from build123d import *

# Parameters (mm, degrees)
SKETCH1_W           = 101.6
SKETCH1_H           = 101.6
SKETCH1_R           = 6.5
SKETCH1_R_2         = 1.5
SKETCH1_R_3         = 3.175
SKETCH1_R_4         = 4
SKETCH1_R_5         = 2.0828
BOSS_EXTRUDE1_DEPTH = 5.9944


with BuildPart() as part:
    # Sketch1 → Boss-Extrude1 (new body)
    with BuildSketch(Plane.XY):
        with Locations((50.8, 50.8)):
            Rectangle(SKETCH1_W, SKETCH1_H)
        with Locations(Location((76.2, 57.8, 0), (0, 0, 180))):
            Circle(SKETCH1_R, mode=Mode.SUBTRACT)
        with Locations(Location((60.7, 50.8, 0), (0, 0, 180))):
            Circle(SKETCH1_R_2, mode=Mode.SUBTRACT)
        with Locations(Location((91.7, 50.8, 0), (0, 0, 180))):
            Circle(SKETCH1_R_2, mode=Mode.SUBTRACT)
        with Locations(Location((83.95, 37.376606241, 0), (0, 0, 180))):
            Circle(SKETCH1_R_2, mode=Mode.SUBTRACT)
        with Locations(Location((68.45, 37.376606241, 0), (0, 0, 180))):
            Circle(SKETCH1_R_2, mode=Mode.SUBTRACT)
        with Locations(Location((68.45, 64.223393759, 0), (0, 0, 180))):
            Circle(SKETCH1_R_2, mode=Mode.SUBTRACT)
        with Locations(Location((83.95, 64.223393759, 0), (0, 0, 180))):
            Circle(SKETCH1_R_2, mode=Mode.SUBTRACT)
        with Locations(Location((12.7, 88.9, 0), (0, 0, 180))):
            Circle(SKETCH1_R_3, mode=Mode.SUBTRACT)
        with Locations(Location((88.9, 88.9, 0), (0, 0, 180))):
            Circle(SKETCH1_R_3, mode=Mode.SUBTRACT)
        with Locations(Location((25.4, 57.8, 0), (0, 0, 180))):
            Circle(SKETCH1_R_4, mode=Mode.SUBTRACT)
        with Locations(Location((15.875, 67.325, 0), (0, 0, 180))):
            Circle(SKETCH1_R_5, mode=Mode.SUBTRACT)
        with Locations(Location((34.925, 67.325, 0), (0, 0, 180))):
            Circle(SKETCH1_R_5, mode=Mode.SUBTRACT)
        with Locations(Location((34.925, 48.275, 0), (0, 0, 180))):
            Circle(SKETCH1_R_5, mode=Mode.SUBTRACT)
        with Locations(Location((15.875, 48.275, 0), (0, 0, 180))):
            Circle(SKETCH1_R_5, mode=Mode.SUBTRACT)
        with Locations(Location((50.8, 88.9, 0), (0, 0, 180))):
            Circle(SKETCH1_R_3, mode=Mode.SUBTRACT)
        with Locations(Location((50.8, 25.4, 0), (0, 0, 180))):
            Circle(SKETCH1_R_3, mode=Mode.SUBTRACT)
        with Locations(Location((50.8, 12.7, 0), (0, 0, 180))):
            Circle(SKETCH1_R_3, mode=Mode.SUBTRACT)
    extrude(amount=BOSS_EXTRUDE1_DEPTH)


solid = part.part
CAD build for the part. Positions are in the model's coordinates, mm. Round coordinates to 2 decimals unless told otherwise and drop trailing zeros. Write each loop counter-clockwise with the first axis right and the second up, starting at its lowest first coordinate (ties: lowest second). Pieces come first, ordered by that corner, then holes. Notation, with made-up numbers: (82.25, -33.5) -> (88.25, -33.5) arc R28 cw to (88.25, -1.5) -> close; hole circle Ø3 at (47, 81). An arc over 180 degrees is marked (long way). Answer as a JSON object with one key per item and string values.
(1) Band-saw the part on D-D, the plane x = 50.8. List the corners of the cut face in (y, z) (3 decimals), then the cut area to 3 significant figures.
Reported:
{"outline": "(0, 0) -> (9.525, 0) -> (9.525, 5.994) -> (0, 5.994) -> close; (15.875, 0) -> (22.225, 0) -> (22.225, 5.994) -> (15.875, 5.994) -> close; (28.575, 0) -> (85.725, 0) -> (85.725, 5.994) -> (28.575, 5.994) -> close; (92.075, 0) -> (101.6, 0) -> (101.6, 5.994) -> (92.075, 5.994) -> close", "area": "495 mm^2"}
(2) Two-plate mould, pull along X, no slides. Class faces 1 (the face through (101.6, 50, 3)), 2 (the face through (50, 52, 5.994)), 3 (the face through (67.76, 38.71, 2.96)), 4 (the face through (32.94, 47.65, 2.96)): +X half, -X half, draft (parallel to the pull), parting line (faces both ways), or undercut.
Reported:
{"face 1": "+X half", "face 2": "draft", "face 3": "undercut", "face 4": "undercut"}
(3) Band-saw the part on C-C, the plane y = 88.9. List the corners of the cut face in (x, z) (3 decimals), then the cut area to 3 significant figures.
Reported:
{"outline": "(0, 0) -> (9.525, 0) -> (9.525, 5.994) -> (0, 5.994) -> close; (15.875, 0) -> (47.625, 0) -> (47.625, 5.994) -> (15.875, 5.994) -> close; (53.975, 0) -> (85.725, 0) -> (85.725, 5.994) -> (53.975, 5.994) -> close; (92.075, 0) -> (101.6, 0) -> (101.6, 5.994) -> (92.075, 5.994) -> close", "area": "495 mm^2"}
(4) Band-saw the part on A-A, the plane y = 25.4. List the corners of the cut face in (x, z) (3 decimals).
Reported:
{"outline": "(0, 0) -> (47.625, 0) -> (47.625, 5.994) -> (0, 5.994) -> close; (53.975, 0) -> (101.6, 0) -> (101.6, 5.994) -> (53.975, 5.994) -> close"}
(5) Pin check, flat tips, straight feed: P1, Ø12, axis at x = 68.5, y = 31, coming from the -Z side; P2, Ø7, axis at x = 25.4, y = 57.8, coming from the +Z side. Stop position of each tip, or through.
Reported:
{"P1": "stops at z = 0", "P2": "passes through"}
(6) Probe probe 1 along X at (y, z) = (60, 0.85); probe 2 along X at (y, z) = (65.5, 3.6); probe 3 along X at (y, z) = (25, 5.6). List the from-to ranges inside material, lowest first. Write a range as [from, to].
Reported:
{"probe 1": "x = [0, 22.06], [28.74, 70.08], [82.32, 101.6]", "probe 2": "x = [0, 14.87], [16.88, 33.92], [35.93, 67.66], [69.24, 83.16], [84.74, 101.6]", "probe 3": "x = [0, 47.65], [53.95, 101.6]"}
(7) Band-saw the part on B-B, the plane x = 76.2. List the corners of the cut face in (y, z), then the cut area to 3 significant figures.
Reported:
{"outline": "(0, 0) -> (51.3, 0) -> (51.3, 5.99) -> (0, 5.99) -> close; (64.3, 0) -> (101.6, 0) -> (101.6, 5.99) -> (64.3, 5.99) -> close", "area": "531 mm^2"}
